Verification items for this drawing (mm, ordinates from the low corner). A direction names the side the tool comes from. Round coordinates to 2 decimals unless told otherwise and drop trailing zeros. Order: outer loops, then holes, each group sorted by start corner. A loop starts at its lowest first (then second) coordinate and runs counter-clockwise, first axis right, second up. Notation, with made-up numbers: (-20.5, -8) - (30.5, -8) arc R26 ccw to (30.5, 19) - close; hole circle Ø5 at (52.5, 77.25). An arc over 180 degrees is marked (long way). Use a Markdown table: item, result. Add a question column.
(1) Access from +Z, -Z, +X, -X, +Y, -Y to the whole of each face (thin tool, end or side, straight path). Record for the marked faces 5 and 6.
(2) Thickness scan on line 1 along Y through (x, z) = (43.5, 11.75); line 2 along X through (y, z) = (3, 3.5). Record the ranges inside material, lowest first. Write a range as [from, to].
(3) Mould release check, pull along Y, two halves, no side actions. Record for the marked faces 1, 2, 3 and 4: released by +Y, released by -Y, zero draft, split by the parting line, or undercut.
(4) Section check C-C on z = 6. Record the boundary of the cut face in (x, y) (3 decimals), then the cut area to 3 significant figures.
(5) Section check A-A on x = 21.5. Record the boundary of the cut face in (y, z), then the cut area to 3 significant figures.
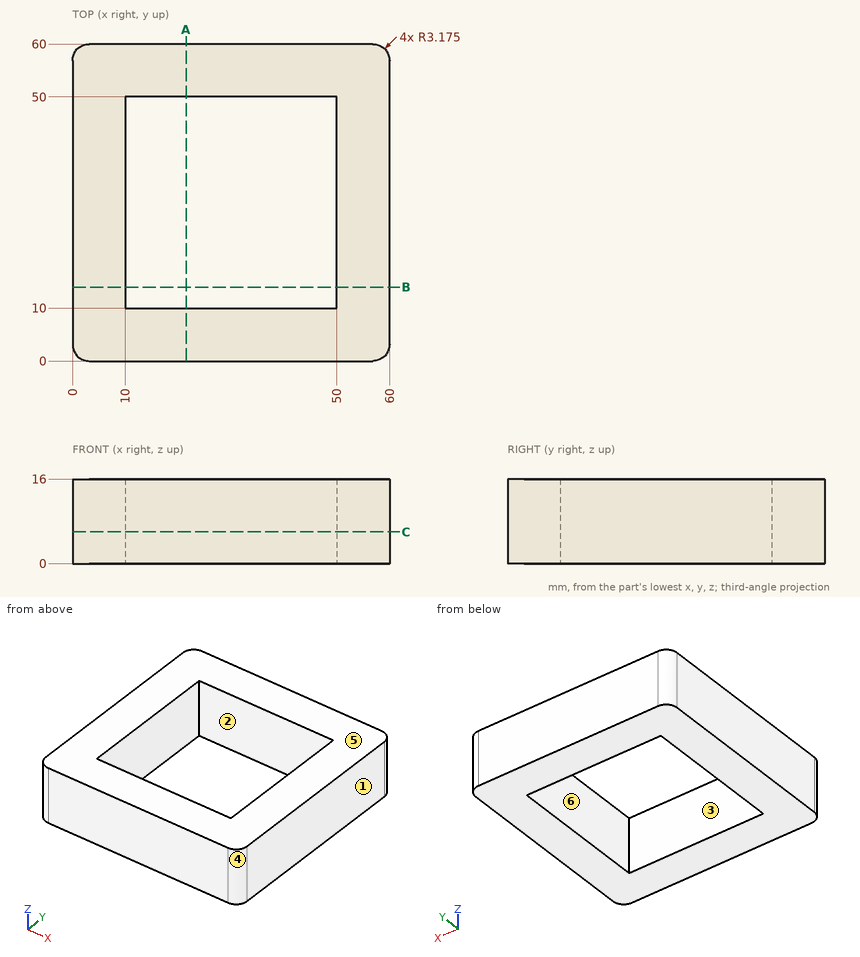
Check sheet entries:
| question | item | result |
|---|---|---|
| 1 | face 5 | +Z, +X, -X, +Y, -Y |
| 1 | face 6 | +Z, -Z |
| 2 | line 1 | y = [0, 10], [50, 60] |
| 2 | line 2 | x = [0, 60] |
| 3 | face 1 | zero draft |
| 3 | face 2 | undercut |
| 3 | face 3 | undercut |
| 3 | face 4 | released by -Y |
| 4 | outline | (0, 3.175) arc R3.175 ccw to (3.175, 0) - (56.825, 0) arc R3.175 ccw to (60, 3.175) - (60, 56.825) arc R3.175 ccw to (56.825, 60) - (3.175, 60) arc R3.175 ccw to (0, 56.825) - close; hole (10, 10) - (50, 10) - (50, 50) - (10, 50) - close |
| 4 | area | 1,990 mm2 |
| 5 | outline | (0, 0) - (10, 0) - (10, 16) - (0, 16) - close; (50, 0) - (60, 0) - (60, 16) - (50, 16) - close |
| 5 | area | 320 mm2 |
